Drawing for the job (mm, zero at the part's lowest x, y, z). A direction names the side the tool comes from. Round coordinates to 2 decimals unless told otherwise and drop trailing zeros. Order: outer loops, then holes, each group sorted by start corner. A loop starts at its lowest first (then second) coordinate and runs counter-clockwise, first axis right, second up. Notation, with made-up numbers: M 69.5,38 L 112.5,38 A30 cw 112.5,65 Z; hole C 72,36 d1. An arc over 180 degrees is marked long. One line per item, written item: value. Start each with the question number.
Item 1: Band-saw the part on D-D, the plane x = 28. Write the cut outline in (y, z).
Item 2: Pin check, flat tips, straight feed: pin 1 (4 mm diameter, centred on x = 23, z = 14, fed in from -Y); pin 2 (3 mm diameter, centred on x = 22, y = 1, fed in from -Z); pin 3 (1 mm diameter, centred on x = 23.5, y = 5.5, fed in from -Z); pin 4 (2 mm diameter, centred on x = 12, y = 2.5, fed in from +Z). Stop position of each tip, or through.
Item 3: Band-saw the part on A-A, the plane x = 15. Write the cut outline in (y, z).
Item 4: Tool access for the marked faces 1 and 2: list every direction of +Z, -Z, +X, -X, +Y, -Y with a clear straight run to the whole face (end or side of a thin tool).
Item 5: Two-plate mould, pull along Z, no slides. Class the marked faces 3, 4 and 5: +Z half, -Z half, draft (parallel to the pull), parting line (faces both ways), or undercut.
Item 6: Band-saw the part on C-C, the plane y = 4.5. Write the cut outline in (x, z), then the cut area to 3 significant figures.
Item 7: Probe L1, parallel to X at y = 3, z = 15; L2, parallel to Z at x = 15, y = 5. List the from-to ranges inside material, lowest first.
Item 8: Band-saw the part on B-B, the plane z = 15. Write the cut outline in (x, y), then the cut area to 3 significant figures.
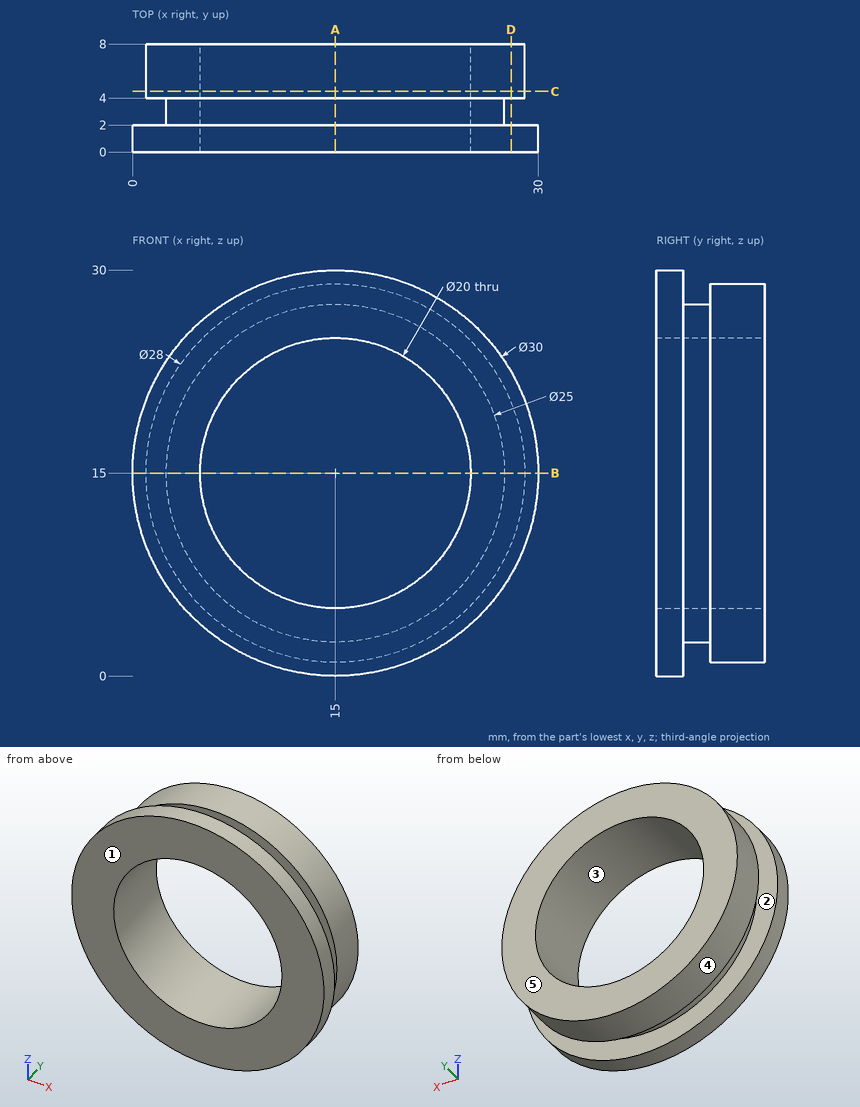
Output:
1. outline: M 0,7.52 L 2,7.52 L 2,22.48 L 0,22.48 Z; M 4,9.8 L 8,9.8 L 8,20.2 L 4,20.2 Z
2. pin 1: stops at y = 0
2. pin 2: stops at z = 1.04
2. pin 3: stops at z = 3.51
2. pin 4: stops at z = 29.85
3. outline: M 0,0 L 2,0 L 2,2.5 L 4,2.5 L 4,1 L 8,1 L 8,5 L 0,5 Z; M 0,25 L 8,25 L 8,29 L 4,29 L 4,27.5 L 2,27.5 L 2,30 L 0,30 Z
4. face 1: +Z, -Z, +X, -X, -Y
4. face 2: none
5. face 3: undercut
5. face 4: parting line
5. face 5: draft
6. outline: C 15,15 d28; hole C 15,15 d20
6. area: 302 mm²
7. L1: x = 2.5 to 5, 25 to 27.5
7. L2: z = 1 to 5, 25 to 29
8. outline: M 0,0 L 5,0 L 5,8 L 1,8 L 1,4 L 2.5,4 L 2.5,2 L 0,2 Z; M 25,0 L 30,0 L 30,2 L 27.5,2 L 27.5,4 L 29,4 L 29,8 L 25,8 Z
8. area: 62.0 mm²
